from build123d import *

# Parameters (mm, degrees)
F0_R     = 28.388449
F1_DEPTH = 90
F2_SIZE  = 2.5
F3_W     = 36.176905
F3_H     = 18.97082
F4_DEPTH = 5


with BuildPart() as f1:
    # F0 (on Front) → F1 (new body)
    with BuildSketch(Plane.XZ):
        Circle(F0_R)
    extrude(amount=F1_DEPTH)

    # F2
    f2_edges = [f1.edges().sort_by_distance(p)[0] for p in [
        (-28.388449, -90, 0),
    ]]
    chamfer(f2_edges, length=F2_SIZE)

    # F3 (on Right) → F4 (cut)
    with BuildSketch(Plane.YZ):
        with Locations((-53.824171, 0)):
            Rectangle(F3_W, F3_H)
    extrude(amount=F4_DEPTH, mode=Mode.SUBTRACT)


solid = f1.part
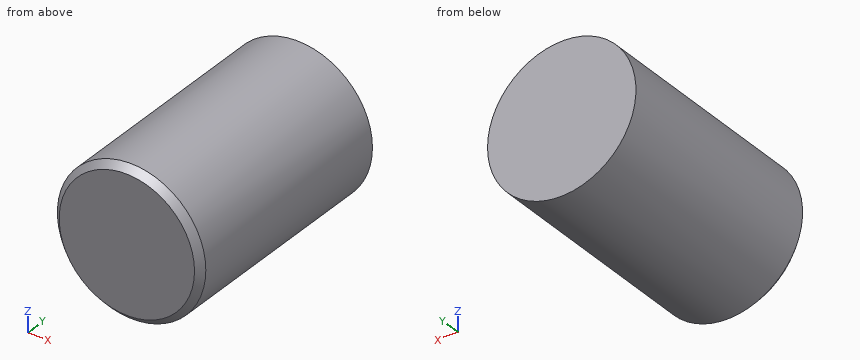
Source: CAD feature listing. Evaluate the final solid. Frame: model axes, mm. Round coordinates to 2 decimals unless told otherwise and drop trailing zeros. Loops run counter-clockwise (first coordinate to the right, second up) from the corner with the lowest first, then second, coordinate; pieces in that order, holes last.
Q1. Ray query, line 1 (Z direction, x = -1, y = -16.5); line 2 (X direction, y = -46.5, z = 7.5); line 3 (X direction, y = -67, z = 8). Return the intervals inside material, ascending.
Q2. Section B-B, the plane y = -29. Return loops of the section in (x, z).
Q3. Section A-A, the plane z = 0. Return loops of the section in (x, y).
Q4. First-contact query: P1, Ø8, axis at x = 8.5, y = -50.5, coming from the +Z side; P2, Ø6, axis at x = 21, y = -58, coming from the -Z side; P3, Ø4, axis at x = 1.5, y = -53.5, coming from the +Z side. Flat tips, straight axial feed; report the tip coordinate or a pass-through.
Solutions:
1. line 1: z = -28.37 to 28.37
1. line 2: x = -27.38 to 0, 5 to 27.38
1. line 3: x = -27.24 to 0, 5 to 27.24
2. outline: circle Ø56.78 at (0, 0)
3. outline: (-28.39, -87.5) - (-25.89, -90) - (25.89, -90) - (28.39, -87.5) - (28.39, 0) - (-28.39, 0) - close; hole (0, -71.91) - (5, -71.91) - (5, -35.74) - (0, -35.74) - close
4. P1: stops at z = 28.03
4. P2: stops at z = -21.95
4. P3: stops at z = 28.39
